CAD build for the part. Positions are in the model's coordinates, mm. A direction names the side the tool comes from. Round coordinates to 2 decimals unless told otherwise and drop trailing zeros. Loops run counter-clockwise (first coordinate to the right, second up) from the corner with the lowest first, then second, coordinate; pieces in that order, holes last.
from build123d import *

# Parameters (mm, degrees)
F0_W     = 79.103634
F0_H     = 79.10363
F0_R     = 22.158127
F0_R_2   = 14.900496
F1_DEPTH = 25.4
F2_DEPTH = 25.4
F3_DEPTH = 25.401


with BuildPart() as f1:
    # F0 (on Front) → F1 (new body)
    with BuildSketch(Plane.XZ):
        with Locations((1.427859, 0.285575)):
            Rectangle(F0_W, F0_H)
        Circle(F0_R, mode=Mode.SUBTRACT)
        Circle(F0_R_2)
        Circle(F0_R)
        Circle(F0_R_2, mode=Mode.SUBTRACT)
    extrude(amount=F1_DEPTH)

    # F0 (on Front) → F2 (join)
    with BuildSketch(Plane.XZ):
        Circle(F0_R)
        Circle(F0_R_2, mode=Mode.SUBTRACT)
    extrude(amount=-F2_DEPTH)

    # F0 (on Front) → F3 (cut, through all)
    with BuildSketch(Plane.XZ):
        Circle(F0_R_2)
    extrude(amount=F3_DEPTH, mode=Mode.SUBTRACT)


solid = f1.part
Item 1: Cut at D-D (x = -33). List the corners of the cut face in (y, z), plus the area to 3 significant figures.
Verdict:
outline: (-25.4, -39.27) - (0, -39.27) - (0, 39.84) - (-25.4, 39.84) - close
area: 2,010 mm2
Item 2: Cut at B-B (z = 0). List the corners of the cut face in (x, y), plus the area to 3 significant figures.
Verdict:
outline: (-38.12, -25.4) - (-14.9, -25.4) - (-14.9, 25.4) - (-22.16, 25.4) - (-22.16, 0) - (-38.12, 0) - close; (14.9, -25.4) - (40.98, -25.4) - (40.98, 0) - (22.16, 0) - (22.16, 25.4) - (14.9, 25.4) - close
area: 1,620 mm2
Item 3: Cut at C-C (y = -20.5). List the corners of the cut face in (x, z).
Verdict:
outline: (-38.12, -39.27) - (40.98, -39.27) - (40.98, 39.84) - (-38.12, 39.84) - close; hole circle Ø29.8 at (0, 0)
Item 4: Flat gauge pins, fed straight in: P1, Ø4, axis at y = 18, z = 15, coming from the +X side; P2, Ø18, axis at x = 0, z = 0, coming from the +Y side; P3, Ø6, axis at x = 28, z = -30.5, coming from the +Y side; P4, Ø5, axis at x = 11, y = 5, coming from the +Z side. Where does each tip first touch, or does it go through?
Verdict:
P1: stops at x = 17.94
P2: passes through
P3: stops at y = 0
P4: stops at z = 20.46
Item 5: Wall check: L1, parallel to Z at x = 0, y = -17.5; L2, parallel to Y at x = -25, z = 24; L3, parallel to Z at x = -8, y = -22. Give the ranges that are in metal, low to high.
Verdict:
L1: z = -39.27 to -14.9, 14.9 to 39.84
L2: y = -25.4 to 0
L3: z = -39.27 to -12.57, 12.57 to 39.84
Item 6: 3-axis set-ups, long thin cutter, end or side, ignore diameter. For faces 1 (the flat face through (-38.124, -13, 0)), 2 (the flat face through (-17, 0, -17)): which of +Z, -Z, +X, -X, +Y, -Y reach the whole face in a straight line?
Verdict:
face 1: +Z, -Z, -X, +Y, -Y
face 2: +Y
Item 7: Cut at A-A (x = 0). List the corners of the cut face in (y, z).
Verdict:
outline: (-25.4, -39.27) - (0, -39.27) - (0, -22.16) - (25.4, -22.16) - (25.4, -14.9) - (-25.4, -14.9) - close; (-25.4, 14.9) - (25.4, 14.9) - (25.4, 22.16) - (0, 22.16) - (0, 39.84) - (-25.4, 39.84) - close
